from build123d import *

# Parameters (mm, degrees)
F0_W          = 58.8
F0_H          = 80.5
F1_DEPTH      = 8
F2_W          = 52.8
F2_H          = 74.5
F3_DEPTH      = 5
F5_R          = 3.5
F6_DEPTH      = 3.5
F9_R          = 1.45
F7_R          = 1.45
F11_DEPTH     = 6.501
F8_R          = 1.45
F12_DEPTH     = 2.5
F10_R         = 1.45
F13_R         = 1.4
F14_W         = 36.8
F14_H         = 3
F15_DEPTH     = 3
F16_W         = 24.6
F16_H         = 3
F17_DEPTH     = 3
F20_DEPTH     = 2
F21_R         = 3
F22_T1_DEPTH  = 5
F22_T3_DEPTH  = 70.5
F22_T5_DEPTH  = 48.8
F22_S9_W      = 2
F22_S9_H      = 2
F22_T10_DEPTH = 2
F22_S15_W     = 2
F22_S15_H     = 2
F22_T16_DEPTH = 2
F22_S21_W     = 2
F22_S21_H     = 2
F22_T22_DEPTH = 2
F22_S27_W     = 2
F22_S27_H     = 2
F22_T28_DEPTH = 2
F23_R         = 2
F24_R         = 1.5
F25_R         = 2
F26_R         = 2.75
F27_DEPTH     = 1.6


# Not quite as in the source:
# - a fillet or chamfer that OpenCascade refuses, or shapes differently, is made with other operations: its cross-section is extruded or revolved along the edge and cut away or added


with BuildPart() as f1:
    # F0 (on Top) → F1 (new body)
    with BuildSketch(Plane.XY):
        with Locations((29.4, 40.25)):
            Rectangle(F0_W, F0_H)
    extrude(amount=F1_DEPTH)

    # F2 (on face) → F3 (cut)
    with BuildSketch(Plane.XY.offset(8)):
        with Locations((29.4, 40.25)):
            Rectangle(F2_W, F2_H)
    extrude(amount=-F3_DEPTH, mode=Mode.SUBTRACT)

    # F5 (on face) → F6 (join)
    with BuildSketch(Plane.XY.offset(3)):
        with Locations((7.75, 7.375)):
            Circle(F5_R)
        with Locations((7.75, 73.125)):
            Circle(F5_R)
        with Locations((51.05, 73.125)):
            Circle(F5_R)
        with Locations((51.05, 7.375)):
            Circle(F5_R)
    extrude(amount=F6_DEPTH)

    # F9 (on face) + F7 (on face) → F11 (cut, through all)
    with BuildSketch(Plane.XY.offset(6.5)):
        with Locations((7.75, 73.125)):
            Circle(F9_R)
    with BuildSketch(Plane.XY.offset(6.5)):
        with Locations((51.05, 7.375)):
            Circle(F7_R)
    extrude(amount=-F11_DEPTH, mode=Mode.SUBTRACT)

    # F8 (on face) → F12 (join)
    with BuildSketch(Plane.XY.offset(6.5)):
        with Locations((51.05, 73.125)):
            Circle(F8_R)
    extrude(amount=F12_DEPTH)

    # F10 (on face) → F12, piece 2 (join)
    with BuildSketch(Plane.XY.offset(6.5)):
        with Locations((7.75, 7.375)):
            Circle(F10_R)
    extrude(amount=F12_DEPTH)

    # F13
    f13_edges = [f1.edges().sort_by_distance(p)[0] for p in [
        (6.3, 7.375, 9),
        (49.6, 73.125, 9),
    ]]
    fillet(f13_edges, radius=F13_R)

    # F14 (on face) → F15 (cut)
    with BuildSketch(Plane.XY.offset(8)):
        with Locations((29.4, 79)):
            Rectangle(F14_W, F14_H)
    extrude(amount=-F15_DEPTH, mode=Mode.SUBTRACT)

    # F16 (on face) → F17 (cut)
    with BuildSketch(Plane.XY.offset(8)):
        with Locations((33.3, 1.5)):
            Rectangle(F16_W, F16_H)
    extrude(amount=-F17_DEPTH, mode=Mode.SUBTRACT)

    # F18 (on face) → F20 (join)
    with BuildSketch(Plane.XY.offset(8)):
        Polygon((47.8, 79), (47.8, 77.5), (55.8, 77.5), (55.8, 3), (45.6, 3), (45.6, 1.5), (57.3, 1.5), (57.3, 79), align=None)
    extrude(amount=F20_DEPTH)

    # F19 (on face) → F20, piece 2 (join)
    with BuildSketch(Plane.XY.offset(8)):
        Polygon((1.5, 1.5), (21, 1.5), (21, 3), (3, 3), (3, 77.5), (11, 77.5), (11, 79), (1.5, 79), align=None)
    extrude(amount=F20_DEPTH)

    # F21
    f21_edges = [f1.edges().sort_by_distance(p)[0] for p in [
        (0, 0, 4),
        (29.4, 0, 0),
        (58.8, 0, 4),
        (0, 40.25, 0),
        (0, 80.5, 4),
        (29.4, 80.5, 0),
        (58.8, 80.5, 4),
        (58.8, 40.25, 0),
    ]]
    fillet(f21_edges, radius=F21_R)

    # F22: fillet of radius 2 on 8 edges, made by hand

    # F22_s2 → F22_t1 (join)
    with BuildSketch(Plane.XY.offset(5)):
        with BuildLine():
            ThreePointArc((53.8, 3), (55.2142135624, 3.5857864376), (55.8, 5))
            Line((55.8, 5), (55.8, 3))
            Line((55.8, 3), (53.8, 3))
        make_face()
        with BuildLine():
            ThreePointArc((5, 3), (3.5857864376, 3.5857864376), (3, 5))
            Line((3, 5), (3, 3))
            Line((3, 3), (5, 3))
        make_face()
        with BuildLine():
            ThreePointArc((5, 77.5), (3.5857864376, 76.9142135624), (3, 75.5))
            Line((3, 75.5), (3, 77.5))
            Line((3, 77.5), (5, 77.5))
        make_face()
        with BuildLine():
            ThreePointArc((53.8, 77.5), (55.2142135624, 76.9142135624), (55.8, 75.5))
            Line((55.8, 75.5), (55.8, 77.5))
            Line((55.8, 77.5), (53.8, 77.5))
        make_face()
    extrude(amount=F22_T1_DEPTH)

    # F22_s4 → F22_t3 (join)
    with BuildSketch(Plane.XZ.offset(-75.5)):
        with BuildLine():
            ThreePointArc((53.8, 3), (55.2142135624, 3.5857864376), (55.8, 5))
            Line((55.8, 5), (55.8, 3))
            Line((55.8, 3), (53.8, 3))
        make_face()
        with BuildLine():
            ThreePointArc((5, 3), (3.5857864376, 3.5857864376), (3, 5))
            Line((3, 5), (3, 3))
            Line((3, 3), (5, 3))
        make_face()
    extrude(amount=F22_T3_DEPTH)

    # F22_s6 → F22_t5 (join)
    with BuildSketch(Plane.YZ.offset(5)):
        with BuildLine():
            ThreePointArc((3, 5), (3.5857864376, 3.5857864376), (5, 3))
            Line((5, 3), (3, 3))
            Line((3, 3), (3, 5))
        make_face()
        with BuildLine():
            ThreePointArc((77.5, 5), (76.9142135624, 3.5857864376), (75.5, 3))
            Line((75.5, 3), (77.5, 3))
            Line((77.5, 3), (77.5, 5))
        make_face()
    extrude(amount=F22_T5_DEPTH)


with BuildPart() as f22_tool8:
    # F22_s9 → F22_t10 (new body)
    with BuildSketch(Plane.XY.offset(5)):
        with Locations((54.8, 4)):
            Rectangle(F22_S9_W, F22_S9_H)
    extrude(amount=-F22_T10_DEPTH)

    # F22_s11 → F22_t12 (revolve, cut)
    with BuildSketch(Plane(origin=(53.8, 5, 5), x_dir=(-0.7071067812, 0.7071067812, 0), z_dir=(-0.7071067812, -0.7071067812, 0))):
        with BuildLine():
            ThreePointArc((0, -2), (2, 0), (0, 2))
            Line((0, 2), (0, -2))
        make_face()
    revolve(axis=Axis((53.8, 5, 5), (0, 0, -1)), mode=Mode.SUBTRACT)


with BuildPart() as f1_1:
    add(f1.part)

    # F22_t7: union F22_tool8
    add(f22_tool8.part)


with BuildPart() as f22_tool14:
    # F22_s15 → F22_t16 (new body)
    with BuildSketch(Plane.XY.offset(5)):
        with Locations((4, 4)):
            Rectangle(F22_S15_W, F22_S15_H)
    extrude(amount=-F22_T16_DEPTH)

    # F22_s17 → F22_t18 (revolve, cut)
    with BuildSketch(Plane(origin=(5, 5, 5), x_dir=(0.7071067812, 0.7071067812, 0), z_dir=(-0.7071067812, 0.7071067812, 0))):
        with BuildLine():
            ThreePointArc((0, -2), (2, 0), (0, 2))
            Line((0, 2), (0, -2))
        make_face()
    revolve(axis=Axis((5, 5, 5), (0, 0, -1)), mode=Mode.SUBTRACT)


with BuildPart() as f1_2:
    add(f1_1.part)

    # F22_t13: union F22_tool14
    add(f22_tool14.part)


with BuildPart() as f22_tool20:
    # F22_s21 → F22_t22 (new body)
    with BuildSketch(Plane.XZ.offset(-75.5)):
        with Locations((4, 4)):
            Rectangle(F22_S21_W, F22_S21_H)
    extrude(amount=-F22_T22_DEPTH)

    # F22_s23 → F22_t24 (revolve, cut)
    with BuildSketch(Plane(origin=(5, 75.5, 5), x_dir=(0.7071067812, 0, 0.7071067812), z_dir=(-0.7071067812, 0, 0.7071067812))):
        with BuildLine():
            ThreePointArc((0, -2), (2, 0), (0, 2))
            Line((0, 2), (0, -2))
        make_face()
    revolve(axis=Axis((5, 75.5, 5), (0, 1, 0)), mode=Mode.SUBTRACT)


with BuildPart() as f1_3:
    add(f1_2.part)

    # F22_t19: union F22_tool20
    add(f22_tool20.part)


with BuildPart() as f22_tool26:
    # F22_s27 → F22_t28 (new body)
    with BuildSketch(Plane.XZ.offset(-75.5)):
        with Locations((54.8, 4)):
            Rectangle(F22_S27_W, F22_S27_H)
    extrude(amount=-F22_T28_DEPTH)

    # F22_s29 → F22_t30 (revolve, cut)
    with BuildSketch(Plane(origin=(53.8, 75.5, 5), x_dir=(-0.7071067812, 0, 0.7071067812), z_dir=(-0.7071067812, 0, -0.7071067812))):
        with BuildLine():
            ThreePointArc((0, -2), (2, 0), (0, 2))
            Line((0, 2), (0, -2))
        make_face()
    revolve(axis=Axis((53.8, 75.5, 5), (0, 1, 0)), mode=Mode.SUBTRACT)


with BuildPart() as f1_4:
    add(f1_3.part)

    # F22_t25: union F22_tool26
    add(f22_tool26.part)

    # F23
    f23_edges = [f1_4.edges().sort_by_distance(p)[0] for p in [
        (57.3, 79, 9),
        (1.5, 79, 9),
        (1.5, 1.5, 9),
        (57.3, 1.5, 9),
    ]]
    fillet(f23_edges, radius=F23_R)

    # F24
    f24_edges = [f1_4.edges().sort_by_distance(p)[0] for p in [
        (11, 79, 5),
        (47.8, 79, 5),
    ]]
    fillet(f24_edges, radius=F24_R)

    # F25
    f25_edges = [f1_4.edges().sort_by_distance(p)[0] for p in [
        (21, 1.5, 5),
        (45.6, 1.5, 5),
    ]]
    fillet(f25_edges, radius=F25_R)

    # F26 (on face) → F27 (cut)
    with BuildSketch(Plane(origin=(0, 0, 0), x_dir=(1, 0, 0), z_dir=(0, 0, -1))):
        with Locations((51.05, -7.375)):
            Circle(F26_R)
        with Locations((7.75, -73.125)):
            Circle(F26_R)
    extrude(amount=-F27_DEPTH, mode=Mode.SUBTRACT)


solid = f1_4.part
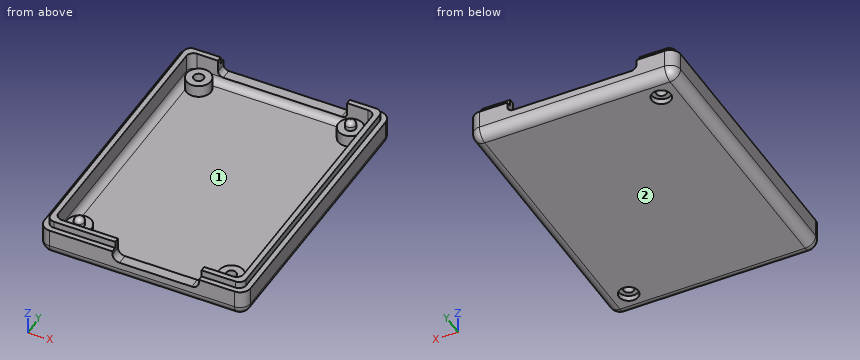
CAD build for the part. Positions are in the model's coordinates, mm. Face numbers are marked on the shaded views. Round coordinates to 2 decimals unless told otherwise and drop trailing zeros. Order: outer loops, then holes, each group sorted by start corner. A loop starts at its lowest first (then second) coordinate and runs counter-clockwise, first axis right, second up. Notation, with made-up numbers: M 2,19 L 58,19 A12 cw 58,29 Z; hole C 80,55 d9. An arc over 180 degrees is marked long. Use one line per item in the form item = value.
Q1. Saw through at A-A on y = 18.5. Give the cut face in (x, z), then the cut area to 3 significant figures.
Recorded:
outline = M 0,3 A3 ccw 3,0 L 55.8,0 A3 ccw 58.8,3 L 58.8,8 L 57.3,8 L 57.3,10 L 55.8,10 L 55.8,5 A2 cw 53.8,3 L 5,3 A2 cw 3,5 L 3,10 L 1.5,10 L 1.5,8 L 0,8 Z
area = 210 mm^2
Q2. Two-plate mould, pull along X, no slides. Class the marked faces 1 and 2: +X half, -X half, draft (parallel to the pull), parting line (faces both ways), or undercut.
Recorded:
face_1 = undercut
face_2 = draft
Q3. Flat gauge pins, fed straight in: P1, Ø1.5, axis at y = 1, z = 8, coming from the +X side; P2, Ø1.5, axis at x = 19.5, z = 6, coming from the +Y side; P3, Ø1.6, axis at x = 53.5, z = 9, coming from the +Y side. Where does each tip first touch, or does it go through?
Recorded:
P1 = 58.53
P2 = 3
P3 = 79
Q4. Probe L1, parallel to Y at x = 51.05, z = 5.35 (3 decimals); L2, parallel to Y at x = 7.75, z = 3.85 (3 decimals); L3, parallel to X at y = 17, z = 8.25. List the from-to ranges inside material, lowest first.
Recorded:
L1 = 0 to 3, 3.875 to 5.925, 8.825 to 10.875, 69.625 to 76.625, 77.5 to 80.5
L2 = 0 to 3.364, 3.875 to 10.875, 69.625 to 71.675, 74.575 to 76.625, 77.136 to 80.5
L3 = 1.5 to 3, 55.8 to 57.3
Q5. Saw through at B-B on x = 26. Give the cut face in (y, z), then the cut area to 3 significant figures.
Recorded:
outline = M 0,3 A3 ccw 3,0 L 77.5,0 A3 ccw 80.5,3 L 80.5,5 L 77.5,5 A2 cw 75.5,3 L 5,3 A2 cw 3,5 L 0,5 Z
area = 251 mm^2
